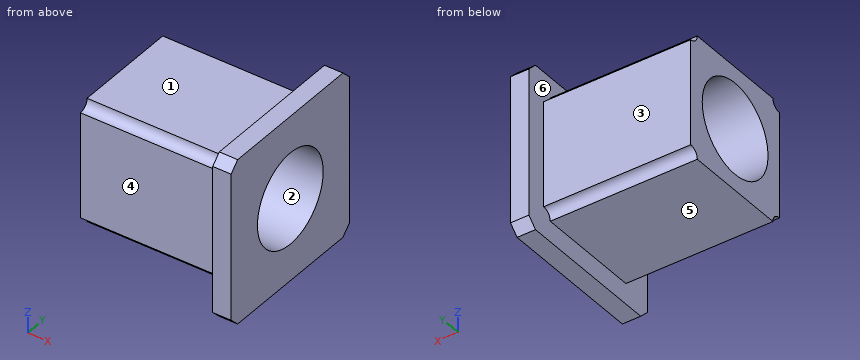
Autodesk Inventor part; units mm, degrees
ref_plane "YZ Plane" through (0, 0, 0) normal (1, 0, 0) x (0, 1, 0)
ref_plane "XZ Plane" through (0, 0, 0) normal (0, 1, 0) x (-1, 0, 0)
ref_plane "XY Plane" through (0, 0, 0) normal (0, 0, 1) x (1, 0, 0)
sketch "Эскиз1" plane through (0, 0, 0) normal (1, 0, 0) x (0, 1, 0)
  line L0 (6.75, 6.75) -> (-6.75, 6.75)
  line L1 (-6.75, 6.75) -> (-6.75, -6.75)
  line L2 (-6.75, -6.75) -> (6.75, -6.75)
  line L3 (6.75, -6.75) -> (6.75, 6.75)
  circle A0 centre (0, 0) radius 5
  dimension "d0" = 13.5
  dimension "d1" = 13.5
  dimension "d2" = 6.75
  dimension "d3" = 6.75
  dimension "d4" = 10
extrude "Выдавливание1" add sketch "Эскиз1" along normal blind 16
ref_plane "РабПлоскость1" through (16, 0, 0) normal (1, 0, 0) x (0, 0, -1)
sketch "Эскиз2" plane through (16, 0, 0) normal (1, 0, 0) x (0, 0, -1)
  line L0 (6.75, -6.75) -> (6.75, 6.75)
  circle A0 centre (6.75, 6.75) radius 1
  line L1 (6.75, 6.75) -> (-6.75, 6.75)
  circle A1 centre (-6.75, 6.75) radius 1
  line L2 (-6.75, -6.75) -> (6.75, -6.75)
  circle A2 centre (-6.75, -6.75) radius 1
  circle A3 centre (6.75, -6.75) radius 1
  point P0 (0, 0)
  dimension "d8" = 2
  dimension "d9" = 2
  dimension "d10" = 2
  dimension "d11" = 2
extrude "Выдавливание2" cut sketch "Эскиз2" against normal blind 16
sketch "Эскиз3" plane through (16, 0, 0) normal (1, 0, 0) x (0, 0, -1)
  line L0 (-9, -9) -> (9, -9)
  line L1 (9, -9) -> (9, 9)
  line L2 (9, 9) -> (-9, 9)
  line L3 (-9, 9) -> (-9, -9)
  line L4 (-9, -9) -> (9, 9) construction
  line L5 (9, -9) -> (-9, 9) construction
  circle A0 centre (0, 0) radius 5
  dimension "d14" = 18
  dimension "d15" = 18
extrude "Выдавливание3" add sketch "Эскиз3" along normal blind 2
chamfer "Фаска1" distance 1 angle 45 4 edges at (17, 9, 9) (17, 9, -9) (17, -9, 9) (17, -9, -9)
properties part number "переходник"
Geometry check sheet. Reference: the model listing, model coordinates, mm. Face numbers are marked on the shaded views. A direction names the side the tool comes from. Coordinates: 2 decimals unless noted, no trailing zeros. Order: outer loops, then holes, each group sorted by start corner. A loop starts at its lowest first (then second) coordinate and runs counter-clockwise, first axis right, second up. Notation, with made-up numbers: (9, 87.25) - (46, 87.25) arc R8 ccw to (46, 95.25) - close; hole circle Ø3 at (19.5, -23.75). An arc over 180 degrees is marked (long way). Answer in a Markdown table with one row per item. Add a question column.
1) Cross-section at C-C, the plane y = -3.5. Record the cut outline in (x, z).
2) Cross-section at D-D, the plane z = -6.25. Record the cut outline in (x, y).
3) Gauge pin test, flat ends, axial feed: P1, Ø3, axis at y = 2.5, z = -7, coming from the -X side; P2, Ø6, axis at x = 2.5, y = 1.5, coming from the +Z side; P3, Ø3.5, axis at x = 5, z = -1.5, coming from the +Y side; P4, Ø5, axis at x = 13, z = -6.5, coming from the -Y side. Record the tip position at first contact, or that the pin passes through.
4) Material ranges on line 1 along Y through (x, z) = (11, 0); line 2 along X through (y, z) = (-7.75, 7), recorded low to high. Write a range as [from, to].
5) Cross-section at B-B, the plane y = 5.5. Record the cut outline in (x, z), then the cut area to 3 significant figures.
6) Set-up check for the marked faces 4, 5 and 6: record each of +Z, -Z, +X, -X, +Y, -Y from which the full face is reachable in a straight line by a thin tool's end or side.
7) Cross-section at A-A, the plane x = 4. Record the cut outline in (y, z).
8) Release check for a two-part mould opening along Z. For the marked faces 1, 2 and 3 record: +Z half, -Z half, draft (parallel to the pull), parting line (faces both ways), or undercut.
Check result:
| question | item | result |
|---|---|---|
| 1 | outline | (0, -6.75) - (16, -6.75) - (16, -9) - (18, -9) - (18, -3.57) - (0, -3.57) - close; (0, 3.57) - (18, 3.57) - (18, 9) - (16, 9) - (16, 6.75) - (0, 6.75) - close |
| 2 | outline | (0, -5.88) - (16, -5.88) - (16, -9) - (18, -9) - (18, 9) - (16, 9) - (16, 5.88) - (0, 5.88) - close |
| 3 | P1 | stops at x = 0 |
| 3 | P2 | stops at z = 6.75 |
| 3 | P3 | stops at y = 6.75 |
| 3 | P4 | stops at y = -6.75 |
| 4 | line 1 | y = [-6.75, -5], [5, 6.75] |
| 4 | line 2 | x = [16, 18] |
| 5 | outline | (0, -6.75) - (16, -6.75) - (16, -9) - (18, -9) - (18, 9) - (16, 9) - (16, 6.75) - (0, 6.75) - close |
| 5 | area | 252 mm² |
| 6 | face 4 | +Z, -Z, -X, -Y |
| 6 | face 5 | -Z, -X, +Y, -Y |
| 6 | face 6 | -X |
| 7 | outline | (-6.75, -5.75) arc R1 cw to (-5.75, -6.75) - (5.75, -6.75) arc R1 cw to (6.75, -5.75) - (6.75, 5.75) arc R1 cw to (5.75, 6.75) - (-5.75, 6.75) arc R1 cw to (-6.75, 5.75) - close; hole circle Ø10 at (0, 0) |
| 8 | face 1 | +Z half |
| 8 | face 2 | undercut |
| 8 | face 3 | draft |
